Source: CAD feature listing. Evaluate the final solid. Frame: model axes, mm. Face numbers are marked on the shaded views. A direction names the side the tool comes from. Give positions to 0.01 mm unless a question says otherwise; leave off trailing zeros. Loops run counter-clockwise (first coordinate to the right, second up) from the corner with the lowest first, then second, coordinate; pieces in that order, holes last. Notation, with made-up numbers: (38.5, -13.5) -> (87.5, -13.5) arc R14 cw to (87.5, 7.5) -> close; hole circle Ø11 at (61.25, 11.25). An arc over 180 degrees is marked (long way). Put each result on its own line as item: value.
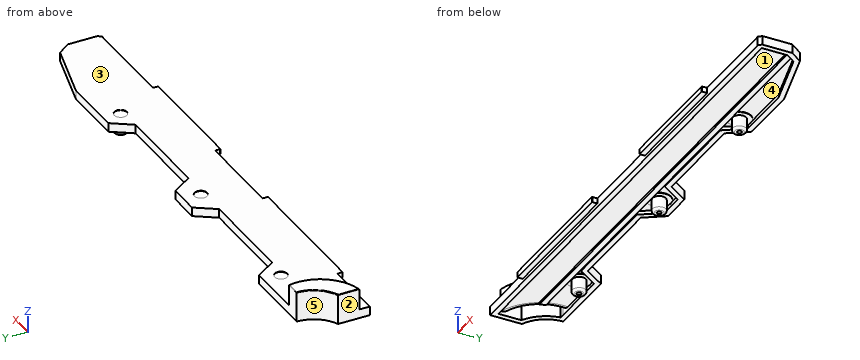
```python
from build123d import *

# Parameters (mm, degrees)
BOSS_EXTRUDE1_DEPTH  = 2
SKETCH6_W            = 31.7
SKETCH6_H            = 1.1999999999999997
BOSS_EXTRUDE2_DEPTH  = 1.2
BOSS_EXTRUDE3_DEPTH  = 1.2
SKETCH4_R            = 1.4099999999999993
SKETCH4_R_2          = 1.4100000000000028
SKETCH4_R_3          = 1.409999999999999
CUT_EXTRUDE6_DEPTH   = 0.1
BOSS_EXTRUDE11_DEPTH = 4.8
SHELL10_DEPTH        = 0.8
SHELL10_START        = 0.8
SHELL10_2_DEPTH      = 4.8
SHELL10_3_OUTLINE_R  = 2.61
SHELL10_3_DEPTH      = 0.7
FILLET2_R            = 2
BOSS_EXTRUDE12_DEPTH = 0.5
SKETCH27_R           = 1.5000000000000042
BOSS_EXTRUDE13_DEPTH = 3
FILLET3_R            = 0.5
SKETCH32_R           = 1.4999999999999973
BOSS_EXTRUDE14_DEPTH = 3
FILLET4_R            = 0.5
SKETCH33_R           = 1.5000000000000009
BOSS_EXTRUDE15_DEPTH = 3
FILLET5_R            = 0.5
SKETCH34_R           = 0.49999999999999917
CUT_EXTRUDE7_DEPTH   = 3
SKETCH35_R           = 0.49999999999999917
CUT_EXTRUDE8_DEPTH   = 3
SKETCH36_R           = 0.49999999999999917
CUT_EXTRUDE9_DEPTH   = 3
FILLET7_R            = 0.1
FILLET8_R            = 0.1
FILLET9_R            = 0.1
FILLET10_R           = 0.1
FILLET11_R           = 0.1


with BuildPart() as part:
    # Sketch1 → Boss-Extrude1 (new body)
    with BuildSketch(Plane.XY):
        with BuildLine():
            Line((0, 0), (113.56, 0))
            Line((113.56, 0), (114.2246801189894, 0.6646806296412225))
            Line((114.2246801189894, 0.6646806296412225), (114.2246801189894, 7.4046806296412235))
            Line((114.2246801189894, 7.4046806296412235), (112.20627968421682, 10.128324324324318))
            Line((112.20627968421682, 10.128324324324318), (98.32468037431536, 13.93))
            Line((98.32468037431536, 13.93), (84.53468037431537, 13.930000000000003))
            Line((84.53468037431537, 13.930000000000003), (81.48697297298213, 9.450000000000003))
            Line((81.48697297298213, 9.450000000000003), (59.046972972982125, 9.450000000000003))
            Line((59.046972972982125, 9.450000000000003), (56.00756633365256, 13.93758367953171))
            Line((56.00756633365256, 13.93758367953171), (49.017566333652546, 13.938836362308603))
            Line((49.017566333652546, 13.938836362308603), (45.980010060525075, 9.450000000000003))
            Line((45.980010060525075, 9.450000000000003), (23.54001006052507, 9.450000000000003))
            Line((23.54001006052507, 9.450000000000003), (20.510017262013168, 13.94394522006733))
            Line((20.510017262013168, 13.94394522006733), (4.610017262013166, 13.946794670160694))
            ThreePointArc((4.610017262013166, 13.946794670160694), (3.3495085223409222, 9.824096158647764), (-8e-17, 7.11))
            Line((-8e-17, 7.11), (0, 0))
        make_face()
    extrude(amount=BOSS_EXTRUDE1_DEPTH)

    # Sketch6 → Boss-Extrude2 (add)
    with BuildSketch(Plane.XZ):
        with Locations((29.68, 1.4000000000000001)):
            Rectangle(SKETCH6_W, SKETCH6_H)
    extrude(amount=BOSS_EXTRUDE2_DEPTH)

    # Sketch7 → Boss-Extrude3 (add)
    with BuildSketch(Plane(origin=(0, 0, 0), x_dir=(-1, 0, 0), z_dir=(0, -1, 0))):
        Polygon((-65.68, -2), (-92.06, -2), (-92.06, -0.8000000000000034), (-65.68, -0.8000000000000002), align=None)
    extrude(amount=BOSS_EXTRUDE3_DEPTH)

    # Sketch4 → Cut-Extrude6 (cut)
    with BuildSketch(Plane.XY.offset(2)):
        with Locations((52.51248680065845, 10.128209973991437)):
            Circle(SKETCH4_R)
        with Locations((18.483506653624264, 10.134308331265466)):
            Circle(SKETCH4_R_2)
        with Locations((86.55081658593453, 10.120000000000001)):
            Circle(SKETCH4_R_3)
    extrude(amount=-CUT_EXTRUDE6_DEPTH, mode=Mode.SUBTRACT)

    # Sketch18 → Boss-Extrude11 (add)
    with BuildSketch(Plane.XY.offset(2)):
        with BuildLine():
            Line((4.610017262013166, 13.946794670160694), (7.8300172620131665, 13.946217611714113))
            ThreePointArc((7.8300172620131665, 13.946217611714113), (6.3125217988837115, 6.53645913408641), (8.7e-16, 2.3700000000000006))
            Line((8.7e-16, 2.3700000000000006), (8.7e-16, 7.110000000000001))
            ThreePointArc((8.7e-16, 7.110000000000001), (3.3495085223409227, 9.824096158647766), (4.610017262013166, 13.946794670160694))
        make_face()
    extrude(amount=BOSS_EXTRUDE11_DEPTH)

    # Shell10: read off the stored shape, not the designer's step
    # Shell10 outline → Shell10 (cut)
    # profile 1 of 4: a face of its own
    with BuildSketch(Plane.XY):
        with BuildLine():
            Line((52.512954541, 12.738209932), (49.654387443, 12.738722218))
            Line((49.654387443, 12.738722218), (46.61690841, 8.25))
            Line((46.61690841, 8.25), (22.901816113, 8.25))
            Line((22.901816113, 8.25), (20.647565145, 11.593400804))
            ThreePointArc((20.647565145, 11.593400804), (20.979532762, 10.89716721), (21.093506654, 10.134308331))
            ThreePointArc((21.093506654, 10.134308331), (16.637792591, 8.288925011), (18.483974394, 12.744308289))
            Line((18.483974394, 12.744308289), (6.783010982, 12.746405227))
            ThreePointArc((6.783010982, 12.746405227), (5.456630529, 7.419449569), (1.2, 3.952918417))
            Line((1.2, 3.952918417), (1.2, 1.2))
            Line((1.2, 1.2), (113.024680119, 1.2))
            Line((113.024680119, 1.2), (113.024680119, 7.008505085))
            Line((113.024680119, 7.008505085), (111.489175152, 9.080526251))
            Line((111.489175152, 9.080526251), (98.163332392, 12.73))
            Line((98.163332392, 12.73), (86.550816586, 12.73))
            ThreePointArc((86.550816586, 12.73), (88.396365285, 11.965548699), (89.160816586, 10.12))
            ThreePointArc((89.160816586, 10.12), (85.782780654, 7.625562026), (84.392831293, 11.588059766))
            Line((84.392831293, 11.588059766), (82.121976504, 8.25))
            Line((82.121976504, 8.25), (58.410391633, 8.25))
            Line((58.410391633, 8.25), (55.37090773, 12.737697756))
            Line((55.37090773, 12.737697756), (52.512954541, 12.738209932))
        make_face()
        with BuildLine():
            ThreePointArc((55.122486801, 10.128209974), (50.666772738, 8.282826654), (52.512954541, 12.738209932))
            ThreePointArc((52.512954541, 12.738209932), (54.358200863, 11.973593294), (55.122486801, 10.128209974))
        make_face(mode=Mode.SUBTRACT)
    # profile 2 of 4: a face of its own
    with BuildSketch(Plane.XY):
        with BuildLine():
            ThreePointArc((18.483974394, 12.744308289), (19.709247434, 12.438578181), (20.647565145, 11.593400804))
            Line((20.647565145, 11.593400804), (19.871746204, 12.744059586))
            Line((19.871746204, 12.744059586), (18.483974394, 12.744308289))
        make_face()
    # profile 3 of 4: a face of its own
    with BuildSketch(Plane.XY):
        with BuildLine():
            Line((85.169683906, 12.73), (84.392831293, 11.588059766))
            ThreePointArc((84.392831293, 11.588059766), (85.330065995, 12.426917422), (86.550816586, 12.73))
            Line((86.550816586, 12.73), (85.169683906, 12.73))
        make_face()
    # profile 4 of 4: a face of its own
    with BuildSketch(Plane.XY):
        with BuildLine():
            ThreePointArc((1.2, 3.952918417), (5.456630529, 7.419449569), (6.783010982, 12.746405227))
            Line((6.783010982, 12.746405227), (5.725437473, 12.746594756))
            ThreePointArc((5.725437473, 12.746594756), (4.237190705, 8.997855303), (1.2, 6.34391511))
            Line((1.2, 6.34391511), (1.2, 3.952918417))
        make_face()
    extrude(amount=SHELL10_DEPTH, mode=Mode.SUBTRACT)

    # Shell10 2 outline → Shell10 2 (cut)
    with BuildSketch(Plane.XY.offset(SHELL10_START)):
        with BuildLine():
            ThreePointArc((1.2, 3.952918417), (5.456630529, 7.419449569), (6.783010982, 12.746405227))
            Line((6.783010982, 12.746405227), (5.725437473, 12.746594756))
            ThreePointArc((5.725437473, 12.746594756), (4.237190705, 8.997855303), (1.2, 6.34391511))
            Line((1.2, 6.34391511), (1.2, 3.952918417))
        make_face()
    extrude(amount=SHELL10_2_DEPTH, mode=Mode.SUBTRACT)

    # Shell10 3 outline → Shell10 3 (cut)
    with BuildSketch(Plane.XY):
        with Locations((52.512486801, 10.128209974)):
            Circle(SHELL10_3_OUTLINE_R)
        with Locations((18.483506654, 10.134308331)):
            Circle(SHELL10_3_OUTLINE_R)
        with Locations((86.550816586, 10.12)):
            Circle(SHELL10_3_OUTLINE_R)
    extrude(amount=SHELL10_3_DEPTH, mode=Mode.SUBTRACT)

    # Fillet2
    fillet2_edges = [part.edges().sort_by_distance(p)[0] for p in [
        (5.456630529005078, 7.419449569008004, 0.8),
    ]]
    fillet(fillet2_edges, radius=FILLET2_R)

    # Sketch19 → Boss-Extrude12 (add)
    with BuildSketch(Plane(origin=(0, 0, 0.8000000000000002), x_dir=(-1, 0, 0), z_dir=(0, 0, -1))):
        with BuildLine():
            Line((-112.10465013060012, 8.250000000000004), (-113.0246801189894, 7.008505084706755))
            Line((-113.0246801189894, 7.008505084706755), (-7.532233645801631, 7.008505084706755))
            ThreePointArc((-7.532233645801631, 7.008505084706755), (-7.836772464238917, 7.620143611633395), (-8.101586568073918, 8.250000000000004))
            Line((-8.101586568073918, 8.250000000000004), (-112.10465013060012, 8.250000000000004))
        make_face()
    extrude(amount=BOSS_EXTRUDE12_DEPTH)

    # Sketch27 → Boss-Extrude13 (add)
    with BuildSketch(Plane(origin=(0, 0, 0.7000000000000001), x_dir=(-1, 0, 0), z_dir=(0, 0, -1))):
        with Locations(Location((-52.51248680065845, 10.128209973991437, 0), (0, 0, 180))):
            Circle(SKETCH27_R)
    extrude(amount=BOSS_EXTRUDE13_DEPTH)

    # Fillet3
    fillet3_edges = [part.edges().sort_by_distance(p)[0] for p in [
        (51.01248680065844, 10.128209973991437, -2.3),
    ]]
    fillet(fillet3_edges, radius=FILLET3_R)

    # Sketch32 → Boss-Extrude14 (add)
    with BuildSketch(Plane(origin=(0, 0, 0.7000000000000001), x_dir=(-1, 0, 0), z_dir=(0, 0, -1))):
        with Locations(Location((-86.55081658593453, 10.120000000000001, 0), (0, 0, 180))):
            Circle(SKETCH32_R)
    extrude(amount=BOSS_EXTRUDE14_DEPTH)

    # Fillet4
    fillet4_edges = [part.edges().sort_by_distance(p)[0] for p in [
        (85.05081658593453, 10.120000000000001, -2.3),
    ]]
    fillet(fillet4_edges, radius=FILLET4_R)

    # Sketch33 → Boss-Extrude15 (add)
    with BuildSketch(Plane(origin=(0, 0, 0.7000000000000001), x_dir=(-1, 0, 0), z_dir=(0, 0, -1))):
        with Locations(Location((-18.483506653624264, 10.134308331265466, 0), (0, 0, 180))):
            Circle(SKETCH33_R)
    extrude(amount=BOSS_EXTRUDE15_DEPTH)

    # Fillet5
    fillet5_edges = [part.edges().sort_by_distance(p)[0] for p in [
        (16.983506653624264, 10.134308331265466, -2.3),
    ]]
    fillet(fillet5_edges, radius=FILLET5_R)

    # Sketch34 → Cut-Extrude7 (cut)
    with BuildSketch(Plane(origin=(0, 0, -2.3), x_dir=(-1, 0, 0), z_dir=(0, 0, -1))):
        with Locations((-52.51248680065845, 10.128209973991437)):
            Circle(SKETCH34_R)
    extrude(amount=-CUT_EXTRUDE7_DEPTH, mode=Mode.SUBTRACT)

    # Sketch35 → Cut-Extrude8 (cut)
    with BuildSketch(Plane(origin=(0, 0, -2.3), x_dir=(-1, 0, 0), z_dir=(0, 0, -1))):
        with Locations((-18.483506653624264, 10.134308331265466)):
            Circle(SKETCH35_R)
    extrude(amount=-CUT_EXTRUDE8_DEPTH, mode=Mode.SUBTRACT)

    # Sketch36 → Cut-Extrude9 (cut)
    with BuildSketch(Plane(origin=(0, 0, -2.3), x_dir=(-1, 0, 0), z_dir=(0, 0, -1))):
        with Locations((-86.55081658593453, 10.120000000000001)):
            Circle(SKETCH36_R)
    extrude(amount=-CUT_EXTRUDE9_DEPTH, mode=Mode.SUBTRACT)

    # Fillet7
    fillet7_edges = [part.edges().sort_by_distance(p)[0] for p in [
        (3.3495085223409236, 9.824096158647766, 6.8),
        (8.7e-16, 4.74, 6.8),
        (6.312521798883712, 6.536459134086408, 6.8),
        (6.220017262013166, 13.946506140937403, 6.8),
    ]]
    fillet(fillet7_edges, radius=FILLET7_R)

    # Fillet8
    fillet8_edges = [part.edges().sort_by_distance(p)[0] for p in [
        (13.83, -1.2, 1.4),
    ]]
    fillet(fillet8_edges, radius=FILLET8_R)

    # Fillet9
    fillet9_edges = [part.edges().sort_by_distance(p)[0] for p in [
        (92.06, -1.2, 1.4000000000000017),
    ]]
    fillet(fillet9_edges, radius=FILLET9_R)

    # Fillet10
    fillet10_edges = [part.edges().sort_by_distance(p)[0] for p in [
        (65.68, -1.2, 1.4),
    ]]
    fillet(fillet10_edges, radius=FILLET10_R)

    # Fillet11
    fillet11_edges = [part.edges().sort_by_distance(p)[0] for p in [
        (45.53, -1.2, 1.4000000000000001),
    ]]
    fillet(fillet11_edges, radius=FILLET11_R)


solid = part.part
```
(1) Line query: probe 1 along X at (y, z) = (10.12, 2.05); probe 2 along Z at (x, y) = (43, 8.75); probe 3 along X at (y, z) = (10, 1.75). Output: solid intervals per line, ascending. Write a range as from..to.
Calculated:
probe 1: x = 3.54..4.91, 6.74..7.81
probe 2: z = 0..2
probe 3: x = 3.46..4.85, 6.86..23.17, 46.35..58.67, 81.86..112.3
(2) First-contact query: P1, Ø1.5, axis at y = 4.5, z = 3.5, coming from the +X side; P2, Ø1.7, axis at x = 18.48, y = 10.13, coming from the -Z side; P3, Ø6, axis at x = 4.5, y = 10, coming from the -Z side; P4, Ø1.4, axis at x = 75, y = 7.5, coming from the -Z side. Flat tips, straight axial feed; report the tip coordinate or a pass-through.
Calculated:
P1: stops at x = 5.28
P2: stops at z = -2.3
P3: stops at z = 0
P4: stops at z = 0.3
(3) Reachability of the marked faces 1 and 2 from +Z, -Z, +X, -X, +Y, -Y: full face, straight path, thin tool, end or side. Return the list, or none.
Calculated:
face 1: -Z
face 2: +Z, -Z, -X, +Y, -Y
(4) Section A-A on z = 4.5. Return loops of the section in (x, y).
Calculated:
outline: (0, 2.37) arc R9.88 ccw to (7.83, 13.95) -> (4.61, 13.95) arc R7.38 cw to (0, 7.11) -> close; hole (1.2, 3.95) arc R8.68 ccw to (6.78, 12.75) -> (5.73, 12.75) arc R8.58 cw to (1.2, 6.34) -> close
(5) Section B-B on x = 34.5. Return loops of the section in (y, z).
Calculated:
outline: (-1.2, 0.8) -> (0, 0.8) -> (0, 0) -> (1.2, 0) -> (1.2, 0.8) -> (7.01, 0.8) -> (7.01, 0.3) -> (8.25, 0.3) -> (8.25, 0) -> (9.45, 0) -> (9.45, 2) -> (-1.2, 2) -> close
(6) Draft query along Y for the marked faces 3, 4 and 5. Return one class per face: released by +Y, released by -Y, zero draft, split by the parting line, or undercut.
Calculated:
face 3: zero draft
face 4: undercut
face 5: released by +Y
